Geometry: final body of the model. Coordinates: model frame, mm. Face numbers are marked on the shaded views. A direction names the side the tool comes from. Round coordinates to 2 decimals unless told otherwise and drop trailing zeros. Order: outer loops, then holes, each group sorted by start corner. A loop starts at its lowest first (then second) coordinate and runs counter-clockwise, first axis right, second up. Notation, with made-up numbers: M 42,-39 L 51,-39 A21 cw 51,-25 Z; hole C -35.5,2 d6. An arc over 180 degrees is marked long. Return JSON: item names as keys, results as strings. Group by question number.
Q1. Cut plane B-B on x = 0. Output: boundary loops of the cut face in (y, z), and give its area (3 significant figures).
Q2. Cut plane A-A on z = 0. Output: boundary loops of the cut face in (x, y), and give its area (3 significant figures).
Q3. Cut plane C-C on y = 6. Output: boundary loops of the cut face in (x, z).
Q4. Cut plane D-D on y = 2.25. Output: boundary loops of the cut face in (x, z).
Q5. Mould query, pull axis Z, two halves, no side actions, for the marked faces 1, 2 and 3. Classes: released by +Z, released by -Z, zero draft, split by the parting line, or undercut.
Q6. Ray query, probe 1 along X at (y, z) = (2.5, 0); probe 2 along X at (y, z) = (5.5, -0.75); probe 3 along X at (y, z) = (0.15, 0). Return the intervals inside material, ascending.
Q7. Access query for the marked faces 4, 5 and 6. Directions: +Z, -Z, +X, -X, +Y, -Y. A direction counts if a zero-diameter tool reaches every point of the face in a straight line with its end or side. Return the directions, or none.
Q8. Contact query for flat-ended pins moving along their axis: pin 1 (3 mm diameter, centred on x = 2.5, y = 4, fed in from -Z); pin 2 (3 mm diameter, centred on y = 5, z = -2, fed in from +X); pin 3 (1 mm diameter, centred on x = 6, z = -0.5, fed in from -Y). Output: stop coordinate, or through.
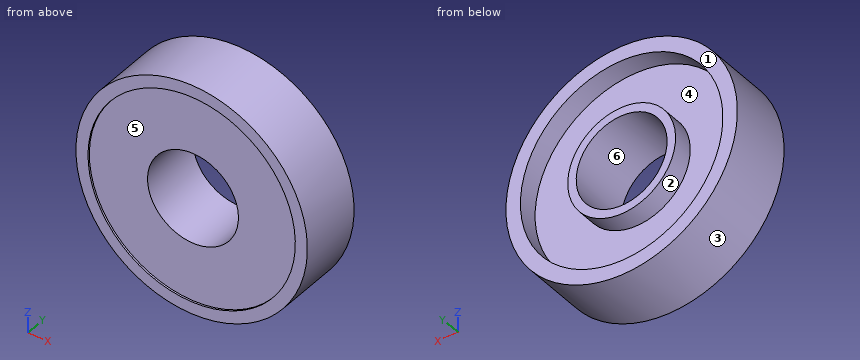
```python
from build123d import *

# Parameters (mm, degrees)
SKETCH1_R           = 12.45
BOSS_EXTRUDE1_DEPTH = 7
SKETCH2_R           = 4.89
CUT_EXTRUDE1_DEPTH  = 19.947427266
SKETCH3_R           = 10.89
SKETCH3_R_2         = 5.8
CUT_EXTRUDE2_DEPTH  = 2.2
SKETCH4_R           = 11.15
CUT_EXTRUDE3_DEPTH  = 0.2


with BuildPart() as part:
    # Sketch1 → Boss-Extrude1 (new body)
    with BuildSketch(Plane(origin=(0, 0, 0), x_dir=(1, 0, 0), z_dir=(0, 1, 0))):
        with Locations(Location((0, 0, 0), (0, 0, 270))):
            Circle(SKETCH1_R)
    extrude(amount=BOSS_EXTRUDE1_DEPTH)

    # Sketch2 → Cut-Extrude1 (cut, through all)
    with BuildSketch(Plane(origin=(0, 7, 0), x_dir=(1, 0, 0), z_dir=(0, 1, 0))):
        with Locations(Location((0, 0, 0), (0, 0, 270))):
            Circle(SKETCH2_R)
    extrude(amount=-CUT_EXTRUDE1_DEPTH, mode=Mode.SUBTRACT)

    # Sketch3 → Cut-Extrude2 (cut)
    with BuildSketch(Plane(origin=(0, 7, 0), x_dir=(1, 0, 0), z_dir=(0, 1, 0))):
        with Locations(Location((0, 0, 0), (0, 0, 270))):
            Circle(SKETCH3_R)
        with Locations(Location((0, 0, 0), (0, 0, 270))):
            Circle(SKETCH3_R_2, mode=Mode.SUBTRACT)
    extrude(amount=-CUT_EXTRUDE2_DEPTH, mode=Mode.SUBTRACT)

    # Sketch4 → Cut-Extrude3 (cut)
    with BuildSketch(Plane.XZ):
        with Locations(Location((0, 0, 0), (0, 0, 270))):
            Circle(SKETCH4_R)
    extrude(amount=-CUT_EXTRUDE3_DEPTH, mode=Mode.SUBTRACT)


solid = part.part
```
Result sheet:
{
 "1": {"outline": "M 0,-12.45 L 7,-12.45 L 7,-10.89 L 4.8,-10.89 L 4.8,-5.8 L 7,-5.8 L 7,-4.89 L 0.2,-4.89 L 0.2,-11.15 L 0,-11.15 Z; M 0,11.15 L 0.2,11.15 L 0.2,4.89 L 7,4.89 L 7,5.8 L 4.8,5.8 L 4.8,10.89 L 7,10.89 L 7,12.45 L 0,12.45 Z", "area": "80.9 mm²"},
 "2": {"outline": "M -12.45,0 L -11.15,0 L -11.15,0.2 L -4.89,0.2 L -4.89,7 L -5.8,7 L -5.8,4.8 L -10.89,4.8 L -10.89,7 L -12.45,7 Z; M 4.89,0.2 L 11.15,0.2 L 11.15,0 L 12.45,0 L 12.45,7 L 10.89,7 L 10.89,4.8 L 5.8,4.8 L 5.8,7 L 4.89,7 Z", "area": "80.9 mm²"},
 "3": {"outline": "C 0,0 d24.9; C 0,0 d11.6; hole C 0,0 d21.78; hole C 0,0 d9.78"},
 "4": {"outline": "C 0,0 d24.9; hole C 0,0 d9.78"},
 "5": {"face 1": "zero draft", "face 2": "undercut", "face 3": "split by the parting line"},
 "6": {"probe 1": "x = -12.45 to -4.89, 4.89 to 12.45", "probe 2": "x = -12.43 to -10.86, -5.75 to -4.83, 4.83 to 5.75, 10.86 to 12.43", "probe 3": "x = -12.45 to -11.15, 11.15 to 12.45"},
 "7": {"face 4": "+Y", "face 5": "-Y", "face 6": "+Y, -Y"},
 "8": {"pin 1": "stops at z = -12.41", "pin 2": "stops at x = 12.44", "pin 3": "stops at y = 0.2"}
}
